Here's how the part is built. I have some questions about the finished solid (model axes, mm). A direction names the side the tool comes from. Round coordinates to 2 decimals unless told otherwise and drop trailing zeros. Loops run counter-clockwise (first coordinate to the right, second up) from the corner with the lowest first, then second, coordinate; pieces in that order, holes last. Notation, with made-up numbers: (21.5, 63) - (53.5, 63) arc R16 cw to (53.5, 83) - close; hole circle Ø4 at (-14, 60). An arc over 180 degrees is marked (long way). Return JSON: item names as keys, results as strings. Group by question number.
```python
from build123d import *

# Parameters (mm, degrees)
EXTRUDE_2_DEPTH      = 20
EXTRUDE_2_DEPTH_BACK = 10
EXTRUDE_1_DEPTH      = 55


with BuildPart() as part:
    # 草图3 → 凸台-拉伸2 (new body, two sides)
    with BuildSketch(Plane.XY) as extrude_2_sk:
        with BuildLine():
            Line((0, 12.5), (100, 12.5))
            ThreePointArc((100, 12.5), (112.5, 0), (100, -12.5))
            Line((100, -12.5), (0, -12.5))
            ThreePointArc((0, -12.5), (-12.5, 0), (0, 12.5))
        make_face()
    extrude(amount=EXTRUDE_2_DEPTH)
    extrude(extrude_2_sk.sketch, amount=-EXTRUDE_2_DEPTH_BACK)

    # 草图4 → 拉伸-薄壁1 (add)
    with BuildSketch(Plane.XY.offset(20)):
        with BuildLine():
            Line((100, 12.5), (0, 12.5))
            ThreePointArc((0, 12.5), (-12.5, 0), (0, -12.5))
            Line((0, -12.5), (100, -12.5))
            ThreePointArc((100, -12.5), (112.5, 0), (100, 12.5))
        make_face()
        with BuildLine():
            Line((100, 7.5), (0, 7.5))
            ThreePointArc((0, 7.5), (-7.5, 0), (0, -7.5))
            Line((0, -7.5), (100, -7.5))
            ThreePointArc((100, -7.5), (107.5, 0), (100, 7.5))
        make_face(mode=Mode.SUBTRACT)
    extrude(amount=EXTRUDE_1_DEPTH)


solid = part.part
```
Q1. Please list where these lines run through material, in increasing order: line 1 (Y direction, x = 55, z = 38.5); line 2 (X direction, y = -5.5, z = 51); line 3 (Z direction, x = 44.5, y = 1.25).
Q2. Will these pins go through, and if not, where does the flat tip stop? pin 1 Ø7.5 at (x, y) = (62.5, 3) entering from +Z; pin 2 Ø1.5 at (y, z) = (8.5, 37.5) entering from -X; pin 3 Ø5 at (y, z) = (-8.5, 56) entering from +X.
Q3. Imagine slicing it at B-B, the plane y = 0. List the corners of the cut face in (x, z) for me, and give its area (3 significant figures).
Q4. Imagine slicing it at C-C, the plane x = 50. List the corners of the cut face in (y, z) for me.
Q5. For faces 1 (the flat face through (49, -12.5, 32)), 2 (the flat face through (51, 7.5, 47)), which set-ups out of +Z, -Z, +X, -X, +Y, -Y let a thin tool reach every point of the face, with its end or its side?
Q6. Imagine slicing it at A-A, the plane z = 53. List the corners of the cut face in (x, y) for me.
Q7. Imagine slicing it at D-D, the plane z = 6.5. List the corners of the cut face in (x, y) for me.
Q8. If we mould it in two halves opening along X, with no side actions, what happens to faces 3 (the cylindrical face through (-12.497, 0.275, 31.905)), 4 (the flat face through (49, 9, 75)), 5 (the cylindrical face through (107.5, -0.16, 47.11))? For each: +X half, -X half, draft (parallel to the pull), parting line (faces both ways), or undercut.
Output values:
{
 "1": {"line 1": "y = -12.5 to -7.5, 7.5 to 12.5", "line 2": "x = -11.22 to -5.1, 105.1 to 111.22", "line 3": "z = -10 to 20"},
 "2": {"pin 1": "stops at z = 20", "pin 2": "stops at x = -9.81", "pin 3": "stops at x = 110.97"},
 "3": {"outline": "(-12.5, -10) - (112.5, -10) - (112.5, 75) - (107.5, 75) - (107.5, 20) - (-7.5, 20) - (-7.5, 75) - (-12.5, 75) - close", "area": "4,300 mm^2"},
 "4": {"outline": "(-12.5, -10) - (12.5, -10) - (12.5, 75) - (7.5, 75) - (7.5, 20) - (-7.5, 20) - (-7.5, 75) - (-12.5, 75) - close"},
 "5": {"face 1": "+Z, -Z, +X, -X, -Y", "face 2": "+Z"},
 "6": {"outline": "(0, -12.5) - (100, -12.5) arc R12.5 ccw to (100, 12.5) - (0, 12.5) arc R12.5 ccw to start; hole (0, -7.5) - (100, -7.5) arc R7.5 ccw to (100, 7.5) - (0, 7.5) arc R7.5 ccw to start"},
 "7": {"outline": "(0, -12.5) - (100, -12.5) arc R12.5 ccw to (100, 12.5) - (0, 12.5) arc R12.5 ccw to start"},
 "8": {"face 3": "-X half", "face 4": "draft", "face 5": "undercut"}
}
